Could you check a few things on this model? Use its own coordinates, in mm. A direction names the side the tool comes from. Round coordinates to 2 decimals unless told otherwise and drop trailing zeros. Loops run counter-clockwise (first coordinate to the right, second up) from the corner with the lowest first, then second, coordinate; pieces in that order, holes last. Notation, with made-up numbers: (26, 41) - (78, 41) arc R30 ccw to (78, 63) - close; hole circle Ø1 at (74.5, 72). An arc over 180 degrees is marked (long way). Put each result on its own line as item: value. Start each with the question number.
Autodesk Inventor part; units mm, degrees
ref_plane "YZ Plane" through (0, 0, 0) normal (1, 0, 0) x (0, 1, 0)
ref_plane "XZ Plane" through (0, 0, 0) normal (0, 1, 0) x (-1, 0, 0)
ref_plane "XY Plane" through (0, 0, 0) normal (0, 0, 1) x (1, 0, 0)
sketch "Skizze1" plane through (0, 0, 0) normal (0, 0, 1) x (1, 0, 0)
  line L0 (-11.9065, 2.1537) -> (13.0935, 2.1537)
  line L1 (13.0935, 2.1537) -> (13.0935, 27.1537)
  line L2 (13.0935, 27.1537) -> (18.0935, 27.1537)
  line L3 (18.0935, 27.1537) -> (18.0935, -2.8463)
  line L4 (18.0935, -2.8463) -> (-11.9065, -2.8463)
  line L5 (-11.9065, -2.8463) -> (-11.9065, 2.1537)
  point P0 (0, 0)
  dimension "d0" = 5
  dimension "d1" = 5
  dimension "d2" = 30
  dimension "d3" = 30
extrude "Extrusion1" add sketch "Skizze1" along normal blind 40
properties part number "Beschlag_camera"
Item 1: Suppose I cut it at C-C, the plane x = 10. List the corners of the cut face in (y, z) for me.
Item 2: Suppose I cut it at A-A, the plane z = 14. List the corners of the cut face in (x, y) for me, then the cut area to 3 significant figures.
Item 3: On a 3-axis mill with a long thin cutter (end or side, diameter ignored), from which of +Z, -Z, +X, -X, +Y, -Y can I reach the whole of each face in a straight line? I mean faces 1 (the face through (16, 27.154, 20)), 2 (the face through (13.094, 14, 20)). Say none if no direction works.
Item 4: Will these pins go through, and if not, where does the flat tip stop? P1, Ø12.5, axis at x = -3.5, z = 10.5, coming from the +Y side; P2, Ø5, axis at y = 14.5, z = 20, coming from the -X side.
Item 5: I need wall thicknesses on line 1 (Y direction, x = 12.75, z = 2); line 2 (X direction, y = 4.25, z = 16.5). Which ranges of each line are inside material? Lowest first, please. Write a range as from..to.
Item 6: Suppose I cut it at B-B, the plane y = 19.75. List the corners of the cut face in (x, z) for me.
Numbers:
1. outline: (-2.85, 0) - (2.15, 0) - (2.15, 40) - (-2.85, 40) - close
2. outline: (-11.91, -2.85) - (18.09, -2.85) - (18.09, 27.15) - (13.09, 27.15) - (13.09, 2.15) - (-11.91, 2.15) - close
2. area: 275 mm^2
3. face 1: +Z, -Z, +X, -X, +Y
3. face 2: +Z, -Z, -X, +Y
4. P1: y = 2.15
4. P2: x = 13.09
5. line 1: -2.85..2.15
5. line 2: 13.09..18.09
6. outline: (13.09, 0) - (18.09, 0) - (18.09, 40) - (13.09, 40) - close
